Source: three-view drawing plus pictorial views. Frame: mm from the lowest corner of the part. Coordinates: 2 decimals unless noted, no trailing zeros. Order: outer loops, then holes, each group sorted by start corner. A loop starts at its lowest first (then second) coordinate and runs counter-clockwise, first axis right, second up. Notation, with made-up numbers: (39.5, -22) -> (78.5, -22) arc R30 ccw to (78.5, 10) -> close; hole circle Ø11 at (84, -33). An arc over 180 degrees is marked (long way). One line per question, with ' | ' between items.
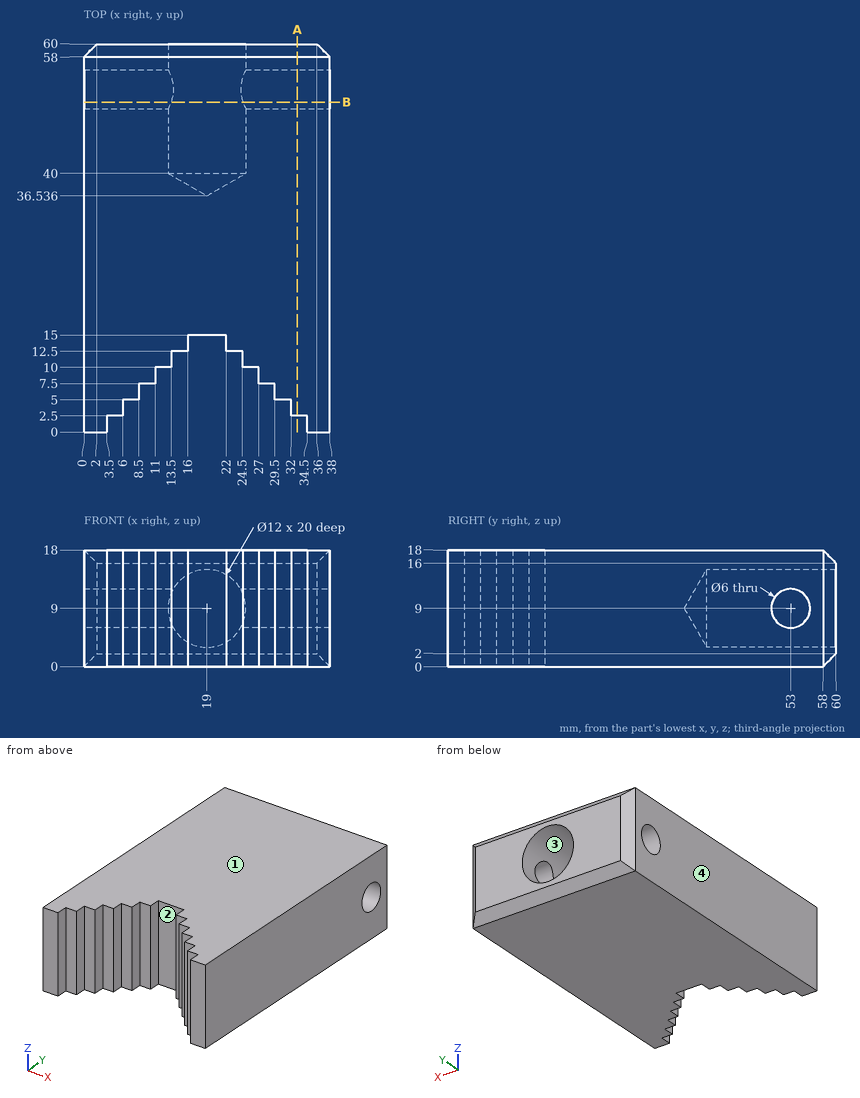
1. Pin query (flat end, axial travel): pin 1 Ø1.2 at (x, z) = (33.5, 7) entering from -Y; pin 2 Ø7 at (x, z) = (19, 9) entering from +Y; pin 3 Ø1.2 at (x, z) = (25.5, 11) entering from -Y. Return the tip coordinate at first contact, or that it passes through.
Recorded:
pin 1: stops at y = 2.5 | pin 2: stops at y = 38.56 | pin 3: stops at y = 10
2. Mould query, pull axis X, two halves, no side actions, for the marked faces 1, 2, 3 and 4. Classes: released by +X, released by -X, zero draft, split by the parting line, or undercut.
Recorded:
face 1: zero draft | face 2: undercut | face 3: undercut | face 4: released by -X
3. Cut plane A-A, the plane x = 33. Return loops of the section in (y, z), and give its area (3 significant figures).
Recorded:
outline: (2.5, 0) -> (58, 0) -> (60, 2) -> (60, 16) -> (58, 18) -> (2.5, 18) -> close; hole circle Ø6 at (53, 9) | area: 1,000 mm^2
4. Cut plane B-B, the plane y = 51. Return loops of the section in (x, z).
Recorded:
outline: (0, 0) -> (38, 0) -> (38, 6.76) -> (24.57, 6.76) arc R6 cw to (13.43, 6.76) -> (0, 6.76) -> close; (0, 11.24) -> (13.43, 11.24) arc R6 cw to (24.57, 11.24) -> (38, 11.24) -> (38, 18) -> (0, 18) -> close
5. Ray query, line 1 (Z direction, x = 19, y = 55); line 2 (Z direction, x = 31, y = 53); line 3 (X direction, y = 45.5, z = 9). Return the intervals inside material, ascending. Write a range as [from, to].
Recorded:
line 1: z = [0, 3], [15, 18] | line 2: z = [0, 6], [12, 18] | line 3: x = [0, 13], [25, 38]
